Check sheet for the modelled part. Datum: model origin and axes. Units: mm. A direction names the side the tool comes from. Round coordinates to 2 decimals unless told otherwise and drop trailing zeros. Loops run counter-clockwise (first coordinate to the right, second up) from the corner with the lowest first, then second, coordinate; pieces in that order, holes last. Notation, with made-up numbers: (-38.5, 58) - (-9.5, 58) arc R8 ccw to (-9.5, 65) - close; hole circle Ø8 at (-20.75, 3.25). An arc over 180 degrees is marked (long way). Put each result on its own line as item: value.
```python
from build123d import *

# Parameters (mm, degrees)
SKETCH2_R           = 1.5
BOSS_EXTRUDE1_DEPTH = 30
CHAMFER1_SIZE       = 0.3
SKETCH6_W           = 3
SKETCH6_H           = 2.75
CUT_EXTRUDE1_DEPTH  = 1.6
SKETCH8_R           = 1.493375673
CUT_EXTRUDE2_DEPTH  = 1
CUT_EXTRUDE2_TAPER  = 45


with BuildPart() as part:
    # Sketch2 → Boss-Extrude1 (new body)
    with BuildSketch(Plane(origin=(0, 0, 0), x_dir=(0, 0, -1), z_dir=(1, 0, 0))):
        Circle(SKETCH2_R)
    extrude(amount=-BOSS_EXTRUDE1_DEPTH)

    # Chamfer1
    chamfer1_edges = [part.edges().sort_by_distance(p)[0] for p in [
        (0, 0, 1.5),
    ]]
    chamfer(chamfer1_edges, length=CHAMFER1_SIZE)

    # Sketch6 → Revolve1 (revolve)
    with BuildSketch(Plane.XY):
        with Locations((-31.5, 1.375)):
            Rectangle(SKETCH6_W, SKETCH6_H)
    revolve(axis=Axis((-30, 0, 0), (1, 0, 0)))

    # Sketch7 → Cut-Extrude1 (cut)
    with BuildSketch(Plane.ZY.offset(33)):
        Polygon((0, 1.443375673), (-1.25, 0.721687836), (-1.25, -0.721687836), (0, -1.443375673), (1.25, -0.721687836), (1.25, 0.721687836), align=None)
    extrude(amount=-CUT_EXTRUDE1_DEPTH, mode=Mode.SUBTRACT)

    # Sketch8 → Cut-Extrude2 (cut)
    with BuildSketch(Plane.ZY.offset(33)):
        Circle(SKETCH8_R)
    extrude(amount=-CUT_EXTRUDE2_DEPTH, taper=CUT_EXTRUDE2_TAPER, mode=Mode.SUBTRACT)


solid = part.part
```
Item 1: Section check B-B on z = 2. Enter the section's corners in (x, y).
Filled sheet:
outline: (-33, -1.89) - (-30, -1.89) - (-30, 1.89) - (-33, 1.89) - close
Item 2: Section check D-D on x = -31. Enter the section's corners in (y, z).
Filled sheet:
outline: circle Ø5.5 at (0, 0)
Item 3: Section check A-A on x = -24.5. Enter the section's corners in (y, z).
Filled sheet:
outline: circle Ø3 at (0, 0)
Item 4: Tool access check on faces 1 (the cylindrical face through (-31.479, -0.596, -2.685)), 2 (the flat face through (-32, 0, -1.25)). Record the directions out of +Z, -Z, +X, -X, +Y, -Y that give a thin tool (end or side, any length) a straight path to the whole face; none if there is none.
Filled sheet:
face 1: +X, -X
face 2: -X
Item 5: Release check for a two-part mould opening along Z. For faces 3 (the cylindrical face through (-14.94, 0.07, 1.5)), 4 (the flat face through (-31.4, 0, 0)), 5 (the flat face through (-30, -1.2, -1.2)) record: +Z half, -Z half, draft (parallel to the pull), parting line (faces both ways), or undercut.
Filled sheet:
face 3: parting line
face 4: undercut
face 5: draft
Item 6: Section check C-C on y = 1.9. Enter the section's corners in (x, z).
Filled sheet:
outline: (-33, -1.99) - (-30, -1.99) - (-30, 1.99) - (-33, 1.99) - close
Item 7: Thickness scan on line 1 (X direction, y = -2.5, z = 0.55); line 2 (X direction, y = -0.25, z = 0); line 3 (Z direction, x = -7, y = 0.1). Record the ranges inside material, lowest first. Write a range as from..to.
Filled sheet:
line 1: -33..-30
line 2: -31.4..0
line 3: -1.5..1.5
Item 8: Go/stop test with flat-tipped pins: pin 1 (2 mm diameter, centred on x = -7, y = 1.5, fed in from -Z); pin 2 (1.5 mm diameter, centred on x = -16.5, z = 1.5, fed in from -Y); pin 3 (1.6 mm diameter, centred on x = -32, y = -0.5, fed in from +Z); pin 4 (1.2 mm diameter, centred on y = 0.5, z = 0, fed in from -X). Record where each tip stops, or that it passes through.
Filled sheet:
pin 1: z = -1.41
pin 2: y = -1.3
pin 3: z = 2.75
pin 4: x = -31.4
